CAD build for the part. Positions are in the model's coordinates, mm. Face numbers are marked on the shaded views. A direction names the side the tool comes from. Round coordinates to 2 decimals unless told otherwise and drop trailing zeros. Write each loop counter-clockwise with the first axis right and the second up, starting at its lowest first coordinate (ties: lowest second). Pieces come first, ordered by that corner, then holes. Notation, with made-up numbers: (12.25, 35.25) -> (47.25, 35.25) arc R24 cw to (47.25, 57.25) -> close; hole circle Ø5 at (21.5, 77.25). An arc over 180 degrees is marked (long way). Put each result on its own line as item: value. Start each with the question number.
1. Saw through at C-C on x = 4. List the corners of the cut face in (y, z).
2. Pull direction Z, two halves, no side cores. Call the marked faces 1, 2 and 3: pulls with the +Z half, pulls with the -Z half, needs draft (parallel to the pull), parting line crosses it, or undercut.
3. 3-axis set-ups, long thin cutter, end or side, ignore diameter. For the marked faces 4 and 5: which of +Z, -Z, +X, -X, +Y, -Y reach the whole face in a straight line?
4. Saw through at B-B on z = -0.75. List the corners of the cut face in (x, y).
5. Drill centre lines: line 1 (X direction, y = 4, z = 1.25); line 2 (X direction, y = 3.25, z = -4.5); line 3 (Z direction, x = -1.5, y = 2.5). Where is each one in solid material? Low to high. Write a range as from..to.
6. Saw through at A-A on y = 2. List the corners of the cut face in (x, z).
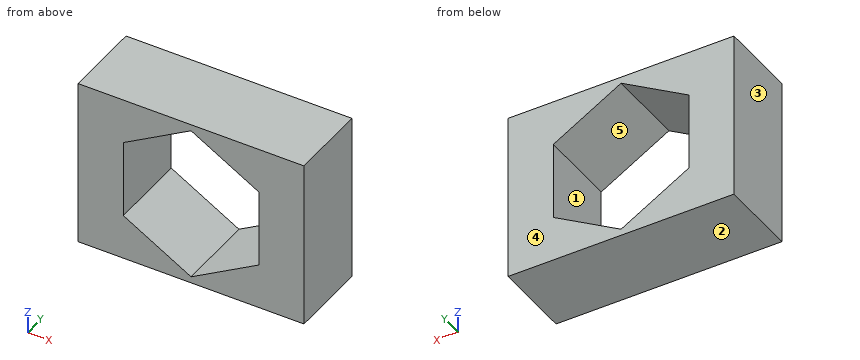
from build123d import *

# Parameters (mm, degrees)
CROQUIS1_W              = 20
CROQUIS1_H              = 15
SALIENTE_EXTRUIR1_DEPTH = 7
CORTAR_EXTRUIR4_DEPTH   = 7


with BuildPart() as part:
    # Croquis1 → Saliente-Extruir1 (new body)
    with BuildSketch(Plane(origin=(0, 0, 0), x_dir=(1, 0, 0), z_dir=(0, 1, 0))):
        Rectangle(CROQUIS1_W, CROQUIS1_H)
    extrude(amount=SALIENTE_EXTRUIR1_DEPTH)

    # Croquis8 → Cortar-Extruir4 (cut)
    with BuildSketch(Plane.XZ):
        Polygon((0, 6.92820323), (-6, 3.464101615), (-6, -3.464101615), (0, -6.92820323), (6, -3.464101615), (6, 3.464101615), align=None)
    extrude(amount=-CORTAR_EXTRUIR4_DEPTH, mode=Mode.SUBTRACT)


solid = part.part
Return value:
1. outline: (0, -7.5) -> (7, -7.5) -> (7, -4.62) -> (0, -4.62) -> close; (0, 4.62) -> (7, 4.62) -> (7, 7.5) -> (0, 7.5) -> close
2. face 1: undercut
2. face 2: pulls with the -Z half
2. face 3: needs draft
3. face 4: +Z, -Z, +X, -X, +Y
3. face 5: +Y, -Y
4. outline: (-10, 0) -> (-6, 0) -> (-6, 7) -> (-10, 7) -> close; (6, 0) -> (10, 0) -> (10, 7) -> (6, 7) -> close
5. line 1: x = -10..-6, 6..10
5. line 2: x = -10..-4.21, 4.21..10
5. line 3: z = -7.5..-6.06, 6.06..7.5
6. outline: (-10, -7.5) -> (10, -7.5) -> (10, 7.5) -> (-10, 7.5) -> close; hole (-6, -3.46) -> (0, -6.93) -> (6, -3.46) -> (6, 3.46) -> (0, 6.93) -> (-6, 3.46) -> close
